from build123d import *

# Parameters (mm, degrees)
SKETCH1_W                      = 45
SKETCH1_H                      = 200
BOSS_EXTRUDE1_DEPTH            = 500
FILLET1_R                      = 4
CUT_EXTRUDE3_DEPTH             = 540.418860697
CUT_EXTRUDE3_DEPTH_BACK        = 540.418860697
CUT_EXTRUDE4_DEPTH             = 540.418860697
CUT_EXTRUDE4_DEPTH_BACK        = 540.418860697
CUT_EXTRUDE5_DEPTH             = 540.418860697
CUT_EXTRUDE5_DEPTH_BACK        = 540.418860697
CUT_EXTRUDE7_DEPTH             = 540.418860697
CUT_EXTRUDE7_DEPTH_BACK        = 540.418860697
F_6_0MM_DOWEL_SLOT_D           = 6
F_6_0MM_DOWEL_SLOT_DEPTH       = 128.197418143
F_6_0MM_DOWEL_SLOT_CSINK_D     = 6.05
F_6_0MM_DOWEL_SLOT_CSINK_ANGLE = 90
F_6_0MM_DOWEL_SLOT_TIP         = 1.802581857


with BuildPart() as part:
    # Sketch1 → Boss-Extrude1 (new body)
    with BuildSketch(Plane.XY):
        with Locations((-8.688255411, 34.272684877)):
            Rectangle(SKETCH1_W, SKETCH1_H)
    extrude(amount=BOSS_EXTRUDE1_DEPTH)

    # Fillet1
    fillet1_edges = [part.edges().sort_by_distance(p)[0] for p in [
        (13.811744589, 134.272684877, 250),
        (13.811744589, -65.727315123, 250),
        (-31.188255411, -65.727315123, 250),
        (-31.188255411, 134.272684877, 250),
    ]]
    fillet(fillet1_edges, radius=FILLET1_R)

    # Sketch4 → Cut-Extrude3 (cut, two sides: drawn at the far end of the back side and taken through both)
    with BuildSketch(Plane(origin=(0, 134.272684877, 0), x_dir=(1, 0, 0), z_dir=(0, 1, 0)).offset(-CUT_EXTRUDE3_DEPTH_BACK)):
        Polygon((-954.529416546, -60.37823327), (-31.188255411, -479.570237952), (13.811744589, -500), (937.152905724, -919.192004683), (98.768896358, -2765.874326953), (-1792.913425912, -1907.060555539), align=None)
    extrude(amount=CUT_EXTRUDE3_DEPTH + CUT_EXTRUDE3_DEPTH_BACK, mode=Mode.SUBTRACT)

    # Sketch5 → Cut-Extrude4 (cut, two sides: drawn at the far end of the back side and taken through both)
    with BuildSketch(Plane(origin=(0, 134.272684877, 0), x_dir=(1, 0, 0), z_dir=(0, 1, 0)).offset(-CUT_EXTRUDE4_DEPTH_BACK)):
        Polygon((781.934937979, 662.017821823), (13.811744589, 0), (-31.188255411, -38.7838855), (-799.311448802, -700.801707323), (-2123.347092448, 835.444679459), (-542.100705666, 2198.264208604), align=None)
    extrude(amount=CUT_EXTRUDE4_DEPTH + CUT_EXTRUDE4_DEPTH_BACK, mode=Mode.SUBTRACT)

    # Sketch6 → Cut-Extrude5 (cut, two sides: drawn at the far end of the back side and taken through both)
    with BuildSketch(Plane(origin=(0, 134.272684877, 0), x_dir=(1, 0, 0), z_dir=(0, 1, 0)).offset(-CUT_EXTRUDE5_DEPTH_BACK)):
        Polygon((-806.445941811, -689.253490297), (-31.188255411, -38.7838855), (13.811744589, -1.027236672), (789.069430988, 649.442368125), (-511.869778607, 2199.957740924), (-2107.385151405, 861.261882502), align=None)
    extrude(amount=CUT_EXTRUDE5_DEPTH + CUT_EXTRUDE5_DEPTH_BACK, mode=Mode.SUBTRACT)

    # Sketch7 → Cut-Extrude7 (cut, two sides: drawn at the far end of the back side and taken through both)
    with BuildSketch(Plane(origin=(0, -65.727315123, 0), x_dir=(-1, 0, 0), z_dir=(0, -1, 0)).offset(-CUT_EXTRUDE7_DEPTH_BACK)):
        Polygon((951.279102129, -47.185095961), (31.188255411, -47.185095961), (-13.811744589, -47.185095961), (-933.902591306, -47.185095961), (-933.902591306, -1887.366789396), (951.279102129, -1887.366789396), align=None)
    extrude(amount=CUT_EXTRUDE7_DEPTH + CUT_EXTRUDE7_DEPTH_BACK, mode=Mode.SUBTRACT)

    # Ø6.0mm Dowel Slot
    with Locations(Plane(origin=(1239.161696342, 134.272684877, 47.185095961), x_dir=(-1, 0, 0), z_dir=(0, 0, 1))):
        with Locations((1247.849951753, 160), (1247.849951753, 100), (1247.849951753, 40)):
            CounterSinkHole(F_6_0MM_DOWEL_SLOT_D / 2, F_6_0MM_DOWEL_SLOT_CSINK_D / 2, depth=F_6_0MM_DOWEL_SLOT_DEPTH, counter_sink_angle=F_6_0MM_DOWEL_SLOT_CSINK_ANGLE)
            with Locations((0, 0, -(F_6_0MM_DOWEL_SLOT_DEPTH + F_6_0MM_DOWEL_SLOT_TIP / 2))):  # 118° drill point
                Cone(0, F_6_0MM_DOWEL_SLOT_D / 2, F_6_0MM_DOWEL_SLOT_TIP, mode=Mode.SUBTRACT)


solid = part.part
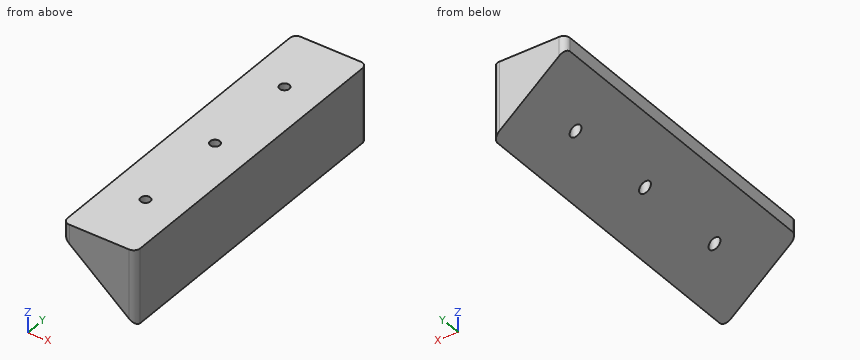
Here's how the part is built. I have some questions about the finished solid (model axes, mm). Coordinates: 2 decimals unless noted, no trailing zeros. Order: outer loops, then holes, each group sorted by start corner. A loop starts at its lowest first (then second) coordinate and runs counter-clockwise, first axis right, second up. Notation, with made-up numbers: (55.5, -22) -> (68.5, -22) arc R34 ccw to (68.5, 11) -> close; hole circle Ø10 at (49.25, -19.75). An arc over 180 degrees is marked (long way). Answer in a Markdown table with one row per item.
(1) I want a section at B-B on z = 15. List the corners of the cut face in (x, y) for me, then the cut area to 3 significant figures.
Answer key:
| item | result |
|---|---|
| outline | (-2.84, -65.73) -> (9.81, -65.73) arc R4 ccw to (13.81, -61.73) -> (13.81, 130.27) arc R4 ccw to (9.81, 134.27) -> (-2.84, 134.27) -> close |
| area | 3,320 mm^2 |
(2) I want a section at C-C on y = 73. List the corners of the cut face in (x, z) for me, then the cut area to 3 significant figures.
Answer key:
| item | result |
|---|---|
| outline | (-31.19, 38.78) -> (13.81, 1.03) -> (13.81, 47.19) -> (-31.19, 47.19) -> close |
| area | 1,230 mm^2 |
(3) Will these pins go through, and if not, where does the flat tip stop? pin 1 Ø5 at (y, z) = (-26.5, 11.5) entering from -X; pin 2 Ø1.5 at (y, z) = (60, 36.5) entering from -X; pin 3 Ø1.5 at (x, y) = (-6.5, -18) entering from -Z.
Answer key:
| item | result |
|---|---|
| pin 1 | x = -1.65 |
| pin 2 | x = -29.36 |
| pin 3 | z = 17.44 |
(4) I want a section at A-A on z = 25.5. List the corners of the cut face in (x, y) for me.
Answer key:
| item | result |
|---|---|
| outline | (-15.36, -65.73) -> (9.81, -65.73) arc R4 ccw to (13.81, -61.73) -> (13.81, 130.27) arc R4 ccw to (9.81, 134.27) -> (-15.36, 134.27) -> close; hole circle Ø6 at (-8.69, -25.73); hole circle Ø6 at (-8.69, 34.27); hole circle Ø6 at (-8.69, 94.27) |
(5) Please list where these lines run through material, in increasing order: probe 1 along Z at (x, y) = (11.5, 13.5); probe 2 along X at (y, z) = (97, 29); probe 3 along Z at (x, y) = (0, 125.5).
Answer key:
| item | result |
|---|---|
| probe 1 | 2.97 to 47.19 |
| probe 2 | -19.53 to -9.94, -7.44 to 13.81 |
| probe 3 | 12.62 to 47.19 |
(6) I want a section at D-D on x = 1.5. List the corners of the cut face in (y, z) for me.
Answer key:
| item | result |
|---|---|
| outline | (-65.73, 11.36) -> (134.27, 11.36) -> (134.27, 47.19) -> (-65.73, 47.19) -> close |
